Check sheet for the modelled part. Datum: model origin and axes. Units: mm. A direction names the side the tool comes from. Coordinates: 2 decimals unless noted, no trailing zeros. Loops run counter-clockwise (first coordinate to the right, second up) from the corner with the lowest first, then second, coordinate; pieces in that order, holes last. Notation, with made-up numbers: M 59,-11.5 L 99,-11.5 A16 cw 99,-0.5 Z; hole C 4.25,5 d6. An arc over 180 degrees is marked long. Answer in a Markdown table with one row per item. Add a question column.
```python
from build123d import *

# Parameters (mm, degrees)
SKETCH1_W           = 228.6
SKETCH1_H           = 88.9
BOSS_EXTRUDE1_DEPTH = 6.35
CUT_EXTRUDE1_DEPTH  = 7.35
LPATTERN1_COUNT     = 2
LPATTERN1_PITCH     = 165.1


with BuildPart() as part:
    # Sketch1 → Boss-Extrude1 (new body)
    with BuildSketch(Plane.XY):
        with Locations((114.3, 44.45)):
            Rectangle(SKETCH1_W, SKETCH1_H)
    extrude(amount=BOSS_EXTRUDE1_DEPTH)

    # Sketch2 → Cut-Extrude1 (cut, through all)
    with BuildSketch(Plane.XY.offset(6.35)):
        with BuildLine():
            Line((23.8125, 76.5937), (39.6875, 76.5937))
            ThreePointArc((39.6875, 76.5937), (46.4312, 69.85), (39.6875, 63.1063))
            Line((39.6875, 63.1063), (23.8125, 63.1063))
            ThreePointArc((23.8125, 63.1063), (17.0688, 69.85), (23.8125, 76.5937))
        make_face()
        with BuildLine():
            Line((23.8125, 25.7937), (39.6875, 25.7937))
            ThreePointArc((39.6875, 25.7937), (46.4312, 19.05), (39.6875, 12.3063))
            Line((39.6875, 12.3063), (23.8125, 12.3063))
            ThreePointArc((23.8125, 12.3063), (17.0688, 19.05), (23.8125, 25.7937))
        make_face()
    cut_extrude1 = extrude(amount=-CUT_EXTRUDE1_DEPTH, mode=Mode.SUBTRACT)

    # LPattern1: Cut-Extrude1 ×2
    with Locations(*[(i * LPATTERN1_PITCH, 0, 0) for i in range(1, LPATTERN1_COUNT)]):
        add(cut_extrude1, mode=Mode.SUBTRACT)


solid = part.part
```
Q1. Mould release check, pull along X, two halves, no side actions. Record for faces 1 (the face through (17.07, 18.9, 3.22)), 2 (the face through (113, 45, 6.35)), 3 (the face through (0, 44, 3)): released by +X, released by -X, zero draft, split by the parting line, or undercut.
Q2. Thickness scan on L1, parallel to Y at x = 199, z = 1.25; L2, parallel to Y at x = 40.5, z = 3.5; L3, parallel to X at y = 17, z = 2.25. Record the ranges inside material, lowest first.
Q3. Cross-section at B-B (x = 194.5). Record the cut outline in (y, z).
Q4. Access from +Z, -Z, +X, -X, +Y, -Y to the whole of each face (thin tool, end or side, straight path). Record for faces 4 (the face through (182.17, 18.9, 3.22)), 5 (the face through (113, 45, 0)).
Q5. Cross-section at A-A (y = 19.05). Record the cut outline in (x, z).
Q6. Go/stop test with a flat-tipped pin: pin 1 (3 mm diameter, centred on x = 198.5, z = 2, fed in from -Y). Record where the tip stops, or that it passes through.
Q7. Cross-section at C-C (z = 3.25). Record the cut outline in (x, y).
Answer key:
| question | item | result |
|---|---|---|
| 1 | face 1 | undercut |
| 1 | face 2 | zero draft |
| 1 | face 3 | released by -X |
| 2 | L1 | 0 to 12.31, 25.79 to 63.11, 76.59 to 88.9 |
| 2 | L2 | 0 to 12.36, 25.74 to 63.16, 76.54 to 88.9 |
| 2 | L3 | 0 to 17.39, 46.11 to 182.49, 211.21 to 228.6 |
| 3 | outline | M 0,0 L 12.31,0 L 12.31,6.35 L 0,6.35 Z; M 25.79,0 L 63.11,0 L 63.11,6.35 L 25.79,6.35 Z; M 76.59,0 L 88.9,0 L 88.9,6.35 L 76.59,6.35 Z |
| 4 | face 4 | +Z, -Z |
| 4 | face 5 | -Z, +X, -X, +Y, -Y |
| 5 | outline | M 0,0 L 17.07,0 L 17.07,6.35 L 0,6.35 Z; M 46.43,0 L 182.17,0 L 182.17,6.35 L 46.43,6.35 Z; M 211.53,0 L 228.6,0 L 228.6,6.35 L 211.53,6.35 Z |
| 6 | pin 1 | y = 0 |
| 7 | outline | M 0,0 L 228.6,0 L 228.6,88.9 L 0,88.9 Z; hole M 23.81,12.31 L 39.69,12.31 A6.74 ccw 39.69,25.79 L 23.81,25.79 A6.74 ccw Z; hole M 23.81,63.11 L 39.69,63.11 A6.74 ccw 39.69,76.59 L 23.81,76.59 A6.74 ccw Z; hole M 188.91,12.31 L 204.79,12.31 A6.74 ccw 204.79,25.79 L 188.91,25.79 A6.74 ccw Z; hole M 188.91,63.11 L 204.79,63.11 A6.74 ccw 204.79,76.59 L 188.91,76.59 A6.74 ccw Z |
